```python
from build123d import *

# Parameters (mm, degrees)
F3_R     = 1.25
F4_DEPTH = 25
F5_SIZE  = 1
F8_DEPTH = 2


with BuildPart() as f1:
    # F0 (on Top) → F1 (revolve)
    with BuildSketch(Plane.XY):
        Polygon((0, 1.25), (0, 2.9657871928), (0, 4), (-1, 4), (-1, 3), (-2, 3), (-2, 4), (-3, 4), (-8, 4), (-13, 4), (-19, 4), (-24, 4), (-25, 4), (-25, 3), (-26, 3), (-26, 4), (-31, 4), (-31, 1), (-27, 1), (-27, 0), (-5, 0), (-5, 1.25), (-0.9906101976, 1.25), align=None)
    revolve(axis=Axis((5.4950757935, 0, 0), (1, 0, 0)))

    # F3 (on offset) → F4 (cut)
    with BuildSketch(Plane.XY.offset(4)):
        with Locations((-21.5, 0)):
            Circle(F3_R)
        with Locations((-10.5, 0)):
            Circle(F3_R)
    extrude(amount=-F4_DEPTH, mode=Mode.SUBTRACT)

    # F5
    f5_edges = [f1.edges().sort_by_distance(p)[0] for p in [
        (0, -1.25, 0),
    ]]
    chamfer(f5_edges, length=F5_SIZE)

    # F7 (on offset) → F8 (cut)
    with BuildSketch(Plane.XZ.offset(-4)):
        with BuildLine():
            Line((-21.5, -1.25), (-10.5, -1.25))
            ThreePointArc((-10.5, -1.25), (-9.25, 0), (-10.5, 1.25))
            Line((-10.5, 1.25), (-21.5, 1.25))
            ThreePointArc((-21.5, 1.25), (-22.75, 0), (-21.5, -1.25))
        make_face()
    extrude(amount=F8_DEPTH, mode=Mode.SUBTRACT)


solid = f1.part
```
Read the model definition and answer for the solid it produces. Units are mm, in the model's axes. A direction names the side the tool comes from. Round coordinates to 2 decimals unless told otherwise and drop trailing zeros. Write each loop counter-clockwise with the first axis right and the second up, starting at its lowest first coordinate (ties: lowest second). Pieces come first, ordered by that corner, then holes. Notation, with made-up numbers: (37.25, -19.5) -> (63.25, -19.5) arc R18 ccw to (63.25, 5.5) -> close; hole circle Ø1 at (-15.75, -18). An arc over 180 degrees is marked (long way). Answer in a Markdown table with one row per item. Add a question column.
1) Consider line 1 (X direction, y = 3, z = 1.5); line 2 (Z direction, x = -1.8, y = 0); line 3 (X direction, y = 0, z = -1.5). Determine where each line is inside the solid, lowest interval first.
2) Find section C-C, the plane y = -3.5. Determine the outline of the cut face in (x, z).
3) Find section A-A, the plane y = 3.5. Determine the outline of the cut face in (x, z), and give its area (3 significant figures).
4) Which of the six approach directions +Z, -Z, +X, -X, +Y, -Y give full straight-line access (tool end or side, diameter ignored) to faces 1 (the face through (-16, 3, -1.25)), 2 (the face through (-2.97, -0.27, -1.22)), 3 (the face through (-27, 0, 0)), 4 (the face through (-26, -1, 3))?
5) Determine the mould class of faces 5 (the face through (-1.5, -3, 0.1)), 6 (the face through (-5, 0, 0)), 7 (the face through (0, -2, -2)) for opening direction Z: pulls with the +Z half, pulls with the -Z half, needs draft (parallel to the pull), parting line crosses it, or undercut.
6) Find section B-B, the plane x = -4. Determine the outline of the cut face in (y, z).
7) Given P1, Ø3, axis at x = -9.5, y = 3, coming from the -Z side; P2, Ø0.8, axis at x = -13.5, z = -0.5, coming from the +Y side; P3, Ø0.6, axis at y = 0, z = 0, coming from the -X side, each flat-ended and moving along its own axis, determine where each tip first touches the part or whether it passes through.
8) Find section D-D, the plane x = -8.5. Determine the outline of the cut face in (y, z).
Findings below:
| question | item | result |
|---|---|---|
| 1 | line 1 | -31 to -26, -25 to -2, -1 to 0 |
| 1 | line 2 | -3 to -1.25, 1.25 to 3 |
| 1 | line 3 | -31 to -22.75, -20.25 to -11.75, -9.25 to -0.75 |
| 2 | outline | (-31, -1.94) -> (-26, -1.94) -> (-26, 1.94) -> (-31, 1.94) -> close; (-25, -1.94) -> (-2, -1.94) -> (-2, 1.94) -> (-25, 1.94) -> close; (-1, -1.94) -> (0, -1.94) -> (0, 1.94) -> (-1, 1.94) -> close |
| 3 | outline | (-31, -1.94) -> (-26, -1.94) -> (-26, 1.94) -> (-31, 1.94) -> close; (-25, -1.94) -> (-2, -1.94) -> (-2, 1.94) -> (-25, 1.94) -> close; (-1, -1.94) -> (0, -1.94) -> (0, 1.94) -> (-1, 1.94) -> close; hole (-21.5, -1.25) -> (-10.5, -1.25) arc R1.25 ccw to (-10.5, 1.25) -> (-21.5, 1.25) arc R1.25 ccw to start |
| 3 | area | 79.9 mm² |
| 4 | face 1 | +Y |
| 4 | face 2 | +X |
| 4 | face 3 | -X |
| 4 | face 4 | none |
| 5 | face 5 | parting line crosses it |
| 5 | face 6 | undercut |
| 5 | face 7 | needs draft |
| 6 | outline | circle Ø8 at (0, 0); hole circle Ø2.5 at (0, 0) |
| 7 | P1 | z = -3.71 |
| 7 | P2 | y = 2 |
| 7 | P3 | x = -27 |
| 8 | outline | circle Ø8 at (0, 0) |
